Autodesk Inventor part; units mm, degrees
ref_plane "YZ Plane" through (0, 0, 0) normal (1, 0, 0) x (0, 1, 0)
ref_plane "XZ Plane" through (0, 0, 0) normal (0, 1, 0) x (-1, 0, 0)
ref_plane "XY Plane" through (0, 0, 0) normal (0, 0, 1) x (1, 0, 0)
sketch "Sketch1" plane through (0, 0, 0) normal (0, 0, 1) x (1, 0, 0)
  line L0 (0, 0) -> (150, 0)
  line L1 (150, 0) -> (150, 60)
  line L2 (150, 60) -> (0, 60)
  line L3 (0, 60) -> (0, 0)
  dimension "d1" = 60
extrude "Extrusion1" add sketch "Sketch1" along normal blind 10
sketch "Sketch2" plane through (0, 0, 0) normal (0, 0, -1) x (-1, 0, 0)
  line L0 (-150, 60) -> (0, 60)
  line L1 (0, 0) -> (-150, 0)
  circle A0 centre (-98.8, 30) radius 5.1
  dimension "d5" = 10.2
  dimension "d6" = 30
  dimension "d20" = 98.8
extrude "Extrusion2" cut sketch "Sketch2" against normal blind 10
sketch "Sketch3" plane through (0, 0, 0) normal (0, 0, -1) x (-1, 0, 0)
  line L0 (-147, 18.65) -> (-147, 41.35) construction
  line L1 (-145.85, 18.65) -> (-145.85, 41.35)
  line L2 (-148.15, 41.35) -> (-148.15, 18.65)
  arc A0 (-148.15, 18.65) -> (-145.85, 18.65) centre (-147, 18.65) ccw
  arc A1 (-145.85, 41.35) -> (-148.15, 41.35) centre (-147, 41.35) ccw
  line L3 (0, 0) -> (-150, 0)
  circle A2 centre (-98.8, 30) radius 5.1
  circle A3 centre (-98.8, 30) radius 5.1
  line L4 (-150, 0) -> (-150, 60)
  line L5 (-150, 60) -> (0, 60)
  line L6 (0, 60) -> (0, 0)
  line L7 (0, 0) -> (-150, 0)
  line L8 (-50.6, 18.65) -> (-50.6, 41.35) construction
  line L9 (-49.45, 18.65) -> (-49.45, 41.35)
  line L10 (-51.75, 41.35) -> (-51.75, 18.65)
  arc A4 (-51.75, 18.65) -> (-49.45, 18.65) centre (-50.6, 18.65) ccw
  arc A5 (-49.45, 41.35) -> (-51.75, 41.35) centre (-50.6, 41.35) ccw
  point P0 (-147, 30)
  point P1 (-147, 42.5)
  point P2 (-147, 17.5)
  point P3 (-50.6, 30)
  point P4 (-50.6, 42.5)
  point P5 (-50.6, 17.5)
  dimension "d10" = 2.3
  dimension "d12" = 25
  dimension "d17" = 3
  dimension "d27" = 2.3
  dimension "d28" = 25
  dimension "d29" = 48.2
extrude "Extrusion3" cut sketch "Sketch3" against normal blind 10 contours A0 L2 A1 L1 | A4 L10 A5 L9
sketch "Sketch4" plane through (0, 0, 10) normal (0, 0, 1) x (1, 0, 0)
  line L0 (0, 60) -> (0, 0)
  line L1 (150, 60) -> (0, 60)
  line L2 (0, 0) -> (43.5504, 0)
  line L3 (43.5504, 0) -> (43.5504, 60)
  line L4 (43.5504, 60) -> (0, 60)
  line L5 (0, 60) -> (0, 0)
extrude "Extrusion4" cut sketch "Sketch4" against normal through all
properties part number "base"
Model file for the job. Use its own axes, mm. A direction names the side the tool comes from. Coordinates: 2 decimals unless noted, no trailing zeros. Order: outer loops, then holes, each group sorted by start corner. A loop starts at its lowest first (then second) coordinate and runs counter-clockwise, first axis right, second up. Notation, with made-up numbers: (-12.75, -27.75) -> (-5.75, -27.75) arc R15 cw to (-5.75, -11.75) -> close; hole circle Ø11 at (70.25, -3). An arc over 180 degrees is marked (long way). Return JSON: item names as keys, results as strings.
Item 1: Wall check: line 1 along X through (y, z) = (41.5, 3); line 2 along Y through (x, z) = (98.8, 5.75); line 3 along X through (y, z) = (31.5, 4). Give the ranges that are in metal, low to high. Write a range as from..to.
Model answer:
{"line 1": "x = 43.55..49.46, 51.74..145.86, 148.14..150", "line 2": "y = 0..24.9, 35.1..60", "line 3": "x = 43.55..49.45, 51.75..93.93, 103.67..145.85, 148.15..150"}
Item 2: Slice it at C-C (z = 5). Write the cut outline in (x, y).
Model answer:
{"outline": "(43.55, 0) -> (150, 0) -> (150, 60) -> (43.55, 60) -> close; hole (49.45, 18.65) arc R1.15 ccw to (51.75, 18.65) -> (51.75, 41.35) arc R1.15 ccw to (49.45, 41.35) -> close; hole circle Ø10.2 at (98.8, 30); hole (145.85, 18.65) arc R1.15 ccw to (148.15, 18.65) -> (148.15, 41.35) arc R1.15 ccw to (145.85, 41.35) -> close"}
Item 3: Slice it at B-B (y = 37). Write the cut outline in (x, z), then the cut area to 3 significant figures.
Model answer:
{"outline": "(43.55, 0) -> (49.45, 0) -> (49.45, 10) -> (43.55, 10) -> close; (51.75, 0) -> (145.85, 0) -> (145.85, 10) -> (51.75, 10) -> close; (148.15, 0) -> (150, 0) -> (150, 10) -> (148.15, 10) -> close", "area": "1,020 mm²"}
Item 4: Slice it at A-A (x = 50.6). Write the cut outline in (y, z), then the cut area to 3 significant figures.
Model answer:
{"outline": "(0, 0) -> (17.5, 0) -> (17.5, 10) -> (0, 10) -> close; (42.5, 0) -> (60, 0) -> (60, 10) -> (42.5, 10) -> close", "area": "350 mm²"}
Item 5: 3-axis set-ups, long thin cutter, end or side, ignore diameter. For faces 1 (the face through (96, 0, 5)), 2 (the face through (49.45, 30, 5)): which of +Z, -Z, +X, -X, +Y, -Y reach the whole face in a straight line?
Model answer:
{"face 1": "+Z, -Z, +X, -X, -Y", "face 2": "+Z, -Z"}
Item 6: Slice it at D-D (y = 30). Write the cut outline in (x, z), then the cut area to 3 significant figures.
Model answer:
{"outline": "(43.55, 0) -> (49.45, 0) -> (49.45, 10) -> (43.55, 10) -> close; (51.75, 0) -> (93.7, 0) -> (93.7, 10) -> (51.75, 10) -> close; (103.9, 0) -> (145.85, 0) -> (145.85, 10) -> (103.9, 10) -> close; (148.15, 0) -> (150, 0) -> (150, 10) -> (148.15, 10) -> close", "area": "916 mm²"}
Item 7: Pin check, flat tip, straight feed: P1, Ø8, axis at x = 98.8, y = 30, coming from the +Z side. Stop position of the tip, or through.
Model answer:
{"P1": "passes through"}
Item 8: Mould opens along X. For faces 3 (the face through (147, 17.5, 4.9)), 4 (the face through (96, 37, 0)), 5 (the face through (43.55, 30, 5)) say: pulls with the +X half, pulls with the -X half, needs draft (parallel to the pull), parting line crosses it, or undercut.
Model answer:
{"face 3": "undercut", "face 4": "needs draft", "face 5": "pulls with the -X half"}
